Can you work these out from the model? Positions are in its coordinate system, mm. Round coordinates to 2 decimals unless told otherwise and drop trailing zeros. Order: outer loops, then holes, each group sorted by start corner. A loop starts at its lowest first (then second) coordinate and runs counter-clockwise, first axis right, second up.
Q1. Will these pins go through, and if not, where does the flat tip stop? P1, Ø12, axis at y = 5.5, z = -81.5, coming from the +X side; P2, Ø2, axis at y = 3, z = 74, coming from the +X side; P3, Ø4, axis at y = 9, z = -45, coming from the +X side; P4, Ø1.5, axis at y = 5.5, z = 60, coming from the +X side.
Q2. If we section it at C-C (z = 45): Please give me the cut outline in (x, y) (3 decimals).
Q3. If I drill on line 1 (X direction, y = -11.75, z = -109); line 2 (Y direction, x = -1, z = -52); line 3 (Z direction, x = 0, y = 13) (3 decimals), over which ranges is the centre line in solid material (lowest first)?
Autodesk Inventor part; units mm, degrees
ref_plane "YZ Plane" through (0, 0, 0) normal (1, 0, 0) x (0, 1, 0)
ref_plane "XZ Plane" through (0, 0, 0) normal (0, 1, 0) x (-1, 0, 0)
ref_plane "XY Plane" through (0, 0, 0) normal (0, 0, 1) x (1, 0, 0)
sketch "Sketch1" plane through (0, 0, 0) normal (0, 0, 1) x (1, 0, 0)
  circle A0 centre (0, 0) radius 14.1986
  dimension "d0" = 28.3972
extrude "Extrusion1" add sketch "Sketch1" along normal mid plane 222.25
sketch "Sketch2" plane through (0, 0, -111.125) normal (0, 0, -1) x (-1, 0, 0)
  arc A0 (4.7625, 6.35) -> (-4.7625, 6.35) centre (0, 0) ccw
  arc A1 (-4.7625, -6.35) -> (4.7625, -6.35) centre (0, 0) ccw
  line L0 (-4.7625, 6.35) -> (-4.7625, -6.35)
  line L1 (4.7625, 6.35) -> (4.7625, -6.35)
  line L2 (4.7625, 0) -> (-4.7625, 0) construction
  dimension "d3" = 9.525
  dimension "d4" = 7.9375
extrude "Extrusion2" add sketch "Sketch2" along normal blind 15.875
sketch "Sketch3" plane through (4.7625, -6.35, -111.125) normal (1, 0, 0) x (0, 0, -1)
  line L0 (15.875, 12.7) -> (15.875, 0) construction
  line L1 (15.875, 6.35) -> (0, 6.35) construction
  line L2 (0, -7.8486) -> (0, 20.5486) construction
  circle A0 centre (9.271, 6.35) radius 3.175
  point P0 (-111.125, 6.35)
  dimension "d7" = 6.604
  dimension "d8" = 6.35
extrude "Extrusion3" cut sketch "Sketch3" against normal through all
sketch "Sketch4" plane through (0, 0, 111.125) normal (0, 0, 1) x (1, 0, 0)
  circle A0 centre (0, 0) radius 7.9375
  dimension "d11" = 15.875
extrude "Extrusion4" add sketch "Sketch4" along normal blind 12.7
chamfer "Chamfer1" distance 1.5875 angle 45 1 edges at (-7.9375, 0, 123.825)
sketch "Sketch5" plane through (0, 0, 123.825) normal (0, 0, 1) x (1, 0, 0)
  circle A0 centre (0, 0) radius 3.175
  dimension "d17" = 6.35
extrude "Extrusion5" cut sketch "Sketch5" against normal blind 152.4
properties part number "cylinder body"
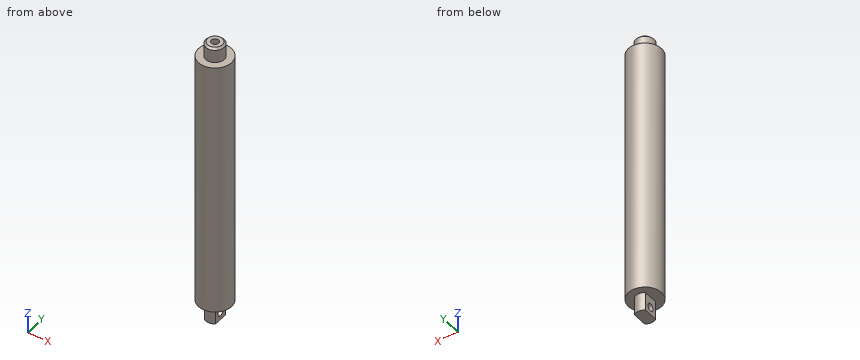
Solution:
1. P1: stops at x = 14.2
1. P2: stops at x = 14.06
1. P3: stops at x = 12.35
1. P4: stops at x = 13.38
2. outline: circle Ø28.397 at (0, 0); hole circle Ø6.35 at (0, 0)
3. line 1: x = -7.97 to 7.97
3. line 2: y = -14.16 to 14.16
3. line 3: z = -111.125 to 111.125
